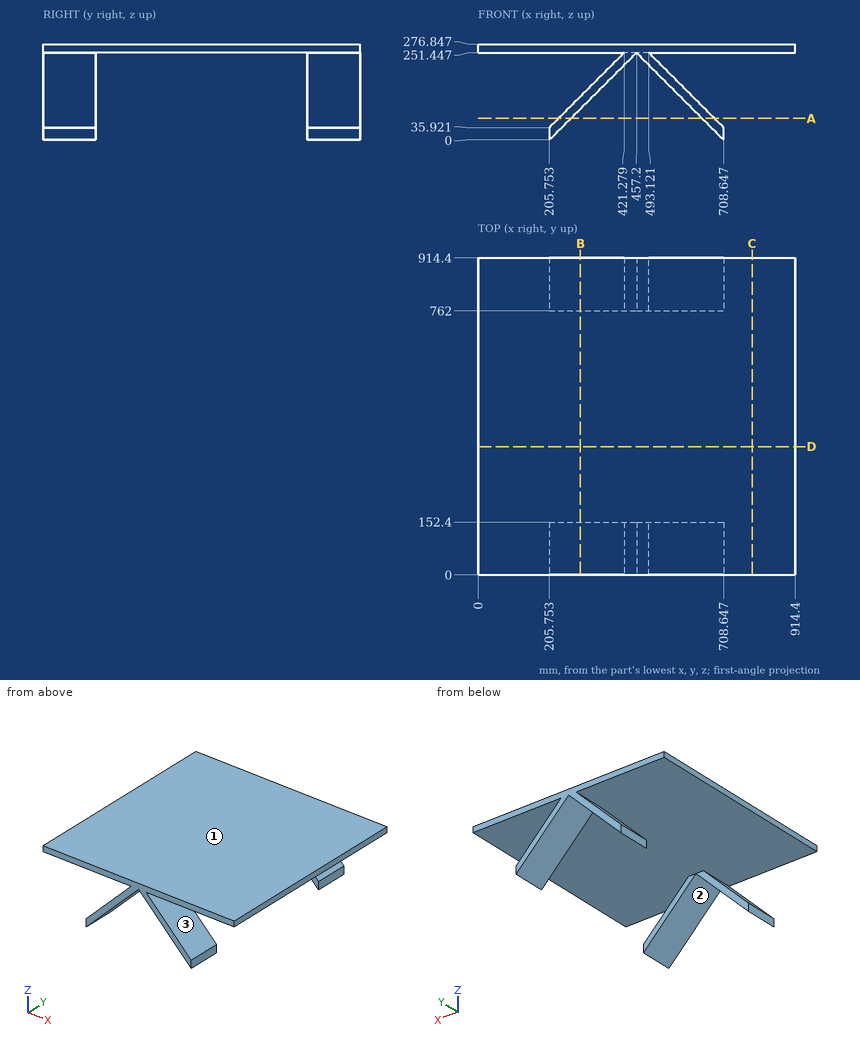
Verification items for this drawing (mm, ordinates from the low corner). Give positions to 0.01 mm unless a question says otherwise; leave off trailing zeros. Write each loop counter-clockwise with the first axis right and the second up, starting at its lowest first coordinate (ties: lowest second). Pieces come first, ordered by that corner, then holes. Notation, with made-up numbers: (48, 71.25) -> (84, 71.25) arc R29 ccw to (84, 102.25) -> close; hole circle Ø7 at (25, 74). An arc over 180 degrees is marked (long way). Write item = value, one per line.
Item 1: Sectioned sample at B-B on x = 295. Record the boundary of the cut face in (y, z).
Output:
outline = (0, 89.25) -> (152.4, 89.25) -> (152.4, 125.17) -> (0, 125.17) -> close; (0, 251.45) -> (914.4, 251.45) -> (914.4, 276.85) -> (0, 276.85) -> close; (762, 89.25) -> (914.4, 89.25) -> (914.4, 125.17) -> (762, 125.17) -> close
Item 2: Release check for a two-part mould opening along Z. For the marked faces 1, 2 and 3 record: +Z half, -Z half, draft (parallel to the pull), parting line (faces both ways), or undercut.
Output:
face_1 = +Z half
face_2 = -Z half
face_3 = undercut
Item 3: Gauge pin test, flat ends, axial feed: pin 1 (6 mm diameter, centred on y = 763.5, z = 234, fed in from +X); pin 2 (1 mm diameter, centred on x = 455, y = 516, fed in from -Z); pin 3 (18 mm diameter, centred on y = 860, z = 16, fed in from +X). Record the tip position at first contact, or that the pin passes through.
Output:
pin_1 = 513.57
pin_2 = 251.45
pin_3 = 708.65
Item 4: Scan lines: probe 1 along Y at (x, z) = (329.5, 142); probe 2 along Z at (x, y) = (783.5, 228); probe 3 along Z at (x, y) = (223.5, 787). Record each from-to range of solid material in increasing order. Write a range as from..to.
Output:
probe_1 = 0..152.4, 762..914.4
probe_2 = 251.45..276.85
probe_3 = 17.75..53.67, 251.45..276.85
Item 5: Sectioned sample at A-A on z = 62. Record the boundary of the cut face in (x, y), and give its area (3 significant figures).
Output:
outline = (231.83, 0) -> (267.75, 0) -> (267.75, 152.4) -> (231.83, 152.4) -> close; (231.83, 762) -> (267.75, 762) -> (267.75, 914.4) -> (231.83, 914.4) -> close; (646.65, 0) -> (682.57, 0) -> (682.57, 152.4) -> (646.65, 152.4) -> close; (646.65, 762) -> (682.57, 762) -> (682.57, 914.4) -> (646.65, 914.4) -> close
area = 21,900 mm^2
Item 6: Sectioned sample at C-C on x = 790.5. Record the boundary of the cut face in (y, z).
Output:
outline = (0, 251.45) -> (914.4, 251.45) -> (914.4, 276.85) -> (0, 276.85) -> close
